```python
from build123d import *


with BuildPart() as f1:
    # F0 (on Front) → F1 (revolve)
    with BuildSketch(Plane.XZ):
        with BuildLine():
            Line((2, -15.170774), (4, -4))
            ThreePointArc((4, -4), (2.828427, -1.171573), (0, 0))
            Line((0, 0), (0, -100))
            Line((0, -100), (9.5, -100))
            Line((9.5, -100), (9.5, -65))
            ThreePointArc((9.5, -65), (8.313642, -62.842418), (6, -62))
            Line((6, -62), (5, -60))
            Line((5, -60), (5, -48))
            Line((5, -48), (7, -42))
            Line((7, -42), (7, -26))
            Line((7, -26), (4.5, -17))
            ThreePointArc((4.5, -17), (3.567458, -15.651518), (2, -15.170774))
        make_face()
    revolve(axis=Axis((0, 0, -50), (0, 0, 1)))


solid = f1.part
```
The model under review builds one solid part; all positions refer to its coordinate system, in mm. A direction names the side the tool comes from. Coordinates: 2 decimals unless noted, no trailing zeros. Loops run counter-clockwise (first coordinate to the right, second up) from the corner with the lowest first, then second, coordinate; pieces in that order, holes last. Notation, with made-up numbers: (-21, 15.5) -> (10, 15.5) arc R3 ccw to (10, 19.5) -> close; hole circle Ø7 at (50.5, -0.5). An arc over 180 degrees is marked (long way). Answer as CSV lines item,"result".
Item 1: Take a section at B-B, the plane z = -91. State the section outline as (x, y) points, and give its area (3 significant figures).
Results below:
outline,"circle Ø19 at (0, 0)"
area,"284 mm2"
Item 2: Insertion check: pin 1 (1.5 mm diameter, centred on y = 1, z = -15, fed in from -X); pin 2 (4 mm diameter, centred on y = -6, z = -19, fed in from +X); pin 3 (5 mm diameter, centred on x = 0, y = 5, fed in from +Z). Each pin has a flat end and moves straight along its axis. Give the tip position at first contact, or say it passes through.
Results below:
pin 1,"stops at x = -3.58"
pin 2,"stops at x = 3.25"
pin 3,"stops at z = -0.88"
Item 3: Take a section at A-A, the plane z = -34. State the section outline as (x, y) points, and give its area (3 significant figures).
Results below:
outline,"circle Ø14 at (0, 0)"
area,"154 mm2"
Item 4: Machinability: for faces 1 (the flat face through (0, 0, -100)), 2 (the cylindrical face through (6.466, -2.681, -33.888)), 3 (the cylindrical face through (-1.08, -4.88, -53.92)), which of the approach directions +Z, -Z, +X, -X, +Y, -Y give a long, thin tool a straight path to every point of the face, cutting with its end or side? Answer none if there is none.
Results below:
face 1,"-Z, +X, -X, +Y, -Y"
face 2,"+Z"
face 3,"none"
Item 5: For L1, parallel to X at y = -3, z = -58; L2, parallel to X at y = -3, z = -90; L3, parallel to Y at x = 4, z = -21.5, list the stretches that pass through material, from the lowest coordinate up.
Results below:
L1,"x = -4 to 4"
L2,"x = -9.01 to 9.01"
L3,"y = -4.13 to 4.13"
Item 6: Draft analysis for pull direction Z (two halves, no side actions). For faces 4 (the conical face through (-2.392, -1.834, -9.507)), 5 (the conical face through (5.203, 1.638, -20.437)), 6 (the cylindrical face through (4.38, -8.43, -82.26)), state which applies: +Z half, -Z half, draft (parallel to the pull), parting line (faces both ways), or undercut.
Results below:
face 4,"undercut"
face 5,"+Z half"
face 6,"draft"
